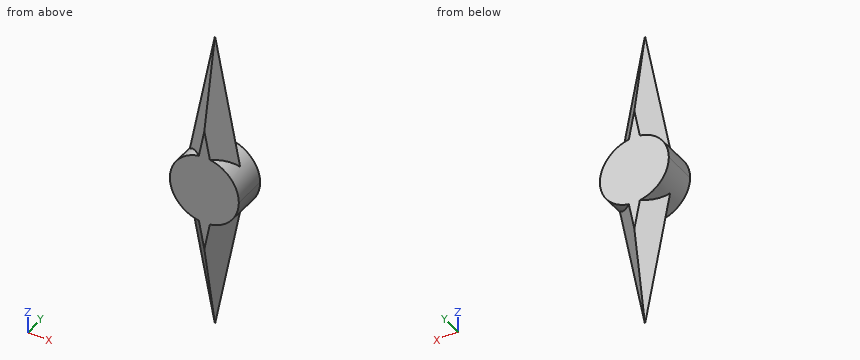
from build123d import *

# Parameters (mm, degrees)
F1_DEPTH = 12.7
F2_SIZE  = 6.34999


# Not quite as in the source:
# - a fillet or chamfer is up to 0.001 mm smaller than in the source, because OpenCascade refuses the exact size


with BuildPart() as f1:
    # F0 (on Front) → F1 (new body)
    with BuildSketch(Plane.XZ):
        with BuildLine():
            Line((0, 0), (12.7, 0))
            ThreePointArc((12.7, 0), (11.8071097568, 4.6778370206), (9.2539906785, 8.6979110436))
            ThreePointArc((9.2539906785, 8.6979110436), (5.0411570967, 11.6566176538), (0, 12.7))
            Line((0, 12.7), (0, 0))
        make_face()
        with BuildLine():
            ThreePointArc((9.2539906785, -8.6979110436), (11.8071097568, -4.6778370206), (12.7, 0))
            Line((12.7, 0), (0, 0))
            Line((0, 0), (0, -12.7))
            ThreePointArc((0, -12.7), (5.0411570967, -11.6566176538), (9.2539906785, -8.6979110436))
        make_face()
        with BuildLine():
            ThreePointArc((0, 12.7), (5.0411570967, 11.6566176538), (9.2539906785, 8.6979110436))
            Line((9.2539906785, 8.6979110436), (0, 55.8542348444))
            Line((0, 55.8542348444), (-9.2539906785, 8.6979110436))
            ThreePointArc((-9.2539906785, 8.6979110436), (-5.0411570967, 11.6566176538), (0, 12.7))
        make_face()
        with BuildLine():
            Line((0, -55.8542348444), (9.2539906785, -8.6979110436))
            ThreePointArc((9.2539906785, -8.6979110436), (5.0411570967, -11.6566176538), (0, -12.7))
            ThreePointArc((0, -12.7), (-5.0411570967, -11.6566176538), (-9.2539906785, -8.6979110436))
            Line((-9.2539906785, -8.6979110436), (0, -55.8542348444))
        make_face()
        with BuildLine():
            Line((-12.7, 0), (0, 0))
            Line((0, 0), (0, 12.7))
            ThreePointArc((0, 12.7), (-5.0411570967, 11.6566176538), (-9.2539906785, 8.6979110436))
            ThreePointArc((-9.2539906785, 8.6979110436), (-11.8071097568, 4.6778370206), (-12.7, 0))
        make_face()
        with BuildLine():
            Line((0, -12.7), (0, 0))
            Line((0, 0), (-12.7, 0))
            ThreePointArc((-12.7, 0), (-11.8071097568, -4.6778370206), (-9.2539906785, -8.6979110436))
            ThreePointArc((-9.2539906785, -8.6979110436), (-5.0411570967, -11.6566176538), (0, -12.7))
        make_face()
    extrude(amount=F1_DEPTH)

    # F2 (size 6.35 in the source; OpenCascade refuses exactly that, so slightly less here)
    f2_edges = [f1.edges().sort_by_distance(p)[0] for p in [
        (4.626995, -12.7, 32.276073),
        (4.626995, 0, 32.276073),
        (-4.626995, -12.7, 32.276073),
        (-4.626995, 0, 32.276073),
        (-4.626995, -12.7, -32.276073),
        (4.626995, -12.7, -32.276073),
        (-4.626995, 0, -32.276073),
        (4.626995, 0, -32.276073),
    ]]
    chamfer(f2_edges, length=F2_SIZE)


solid = f1.part
The model under review builds one solid part; all positions refer to its coordinate system, in mm. Round coordinates to 2 decimals unless told otherwise and drop trailing zeros. Loops run counter-clockwise (first coordinate to the right, second up) from the corner with the lowest first, then second, coordinate; pieces in that order, holes last. Notation, with made-up numbers: (75.5, -38.75) -> (90.5, -38.75) arc R32 cw to (90.5, -11.75) -> close; hole circle Ø8 at (-28, 87). An arc over 180 degrees is marked (long way). Answer as CSV lines item,"result".
1) Add section A-A on y = -10.75. Write out the cut boundary in (x, z), plus the area to 3 significant figures.
Geometry results:
outline,"(-4.12, -12.01) -> (0, -33.01) -> (4.12, -12.01) arc R12.7 ccw to (4.12, 12.01) -> (0, 33.01) -> (-4.12, 12.01) arc R12.7 ccw to start"
area,"672 mm²"
2) To check wall thickness, follow line 1 along Y through (x, z) = (1.25, -19); line 2 along Y through (x, z) = (1, 43.5); line 3 along Z through (x, y) = (-9.5, -11). State the ranges of each line that lie inside material, in increasing order. Write a range as from..to.
Geometry results:
line 1,"y = -12.22..-0.48"
line 2,"y = -7.75..-4.95"
line 3,"z = -8.43..8.43"
3) For P1, Ø1.5, axis at y = -8, z = 18.5, coming from the -X side; P2, Ø4, axis at x = 0.5, y = -5, coming from the +Z side; P3, Ø3, axis at x = -4.5, z = -16.5, coming from the +Y side; P4, Ø6, axis at y = -2, z = -19.5, coming from the +X side, all flat-tipped, find the tip position at first contact; note any pin that passes through.
Geometry results:
P1,"stops at x = -6.43"
P2,"stops at z = 55.85"
P3,"stops at y = -1.69"
P4,"stops at x = 5.81"
